from build123d import *

# Parameters (mm, degrees)
F0_W      = 75
F0_H      = 70
F0_R      = 3.3
F0_W_2    = 30
F0_H_2    = 13.5
F1_DEPTH  = 5
F2_W      = 4
F2_H      = 70
F3_DEPTH  = 55
F4_R      = 19
F4_R_2    = 2.25
F5_DEPTH  = 4
F7_W      = 65.0362595889
F7_H      = 5
F9_R      = 5
F10_DEPTH = 10
F11_R     = 6


with BuildPart() as f1:
    # F0 (on Front) → F1 (new body)
    with BuildSketch(Plane.XZ):
        Rectangle(F0_W, F0_H)
        with Locations((-31.5, -23)):
            Circle(F0_R, mode=Mode.SUBTRACT)
        with Locations((-18.5, -23)):
            Circle(F0_R, mode=Mode.SUBTRACT)
        with Locations((4.5, -10.75)):
            Rectangle(F0_W_2, F0_H_2, mode=Mode.SUBTRACT)
        with Locations((-31.5, 23)):
            Circle(F0_R, mode=Mode.SUBTRACT)
        with Locations((-18.5, 23)):
            Circle(F0_R, mode=Mode.SUBTRACT)
        with Locations((4.5, 10.75)):
            Rectangle(F0_W_2, F0_H_2, mode=Mode.SUBTRACT)
    extrude(amount=F1_DEPTH)

    # F2 (on face) → F3 (join)
    with BuildSketch(Plane.XZ.offset(5)):
        with Locations((35.5, 0)):
            Rectangle(F2_W, F2_H)
    extrude(amount=F3_DEPTH)

    # F4 (on face) → F5 (cut, through all)
    with BuildSketch(Plane.YZ.offset(37.5)):
        with Locations((-30, 0)):
            Circle(F4_R)
        with Locations((-53.5, 23.5)):
            Circle(F4_R_2)
        with Locations((-6.5, 23.5)):
            Circle(F4_R_2)
        with Locations((-6.5, -23.5)):
            Circle(F4_R_2)
        with Locations((-53.5, -23.5)):
            Circle(F4_R_2)
    extrude(amount=-F5_DEPTH, mode=Mode.SUBTRACT)

    # F7 (on line) → F8 (join, up to the next surface of F1)
    with BuildSketch(Plane(origin=(-7.3353011104, -6.1550484563, 0), x_dir=(0.6427876097, -0.7660444431, 0), z_dir=(-0.7660444431, -0.6427876097, 0))):
        with Locations((31.01032112, 32.5)):
            Rectangle(F7_W, F7_H)
        with Locations((31.01032112, -32.5)):
            Rectangle(F7_W, F7_H)
    extrude(until=Until.NEXT, dir=(0.7660444431, 0.6427876097, 0))

    # F9 (on face) → F10 (cut)
    with BuildSketch(Plane(origin=(33.5, 0, 0), x_dir=(0, -1, 0), z_dir=(-1, 0, 0))):
        with Locations((6.5, 23.5000000002)):
            Circle(F9_R)
        with Locations((6.5, -23.4999999998)):
            Circle(F9_R)
    extrude(amount=F10_DEPTH, mode=Mode.SUBTRACT)

    # F11
    f11_edges = [f1.edges().sort_by_distance(p)[0] for p in [
        (-10.5, -2.5, 17.5),
        (19.5, -2.5, 17.5),
        (19.5, -2.5, 4),
        (-10.5, -2.5, 4),
        (19.5, -2.5, -4),
        (19.5, -2.5, -17.5),
        (-10.5, -2.5, -17.5),
        (-10.5, -2.5, -4),
    ]]
    fillet(f11_edges, radius=F11_R)


solid = f1.part
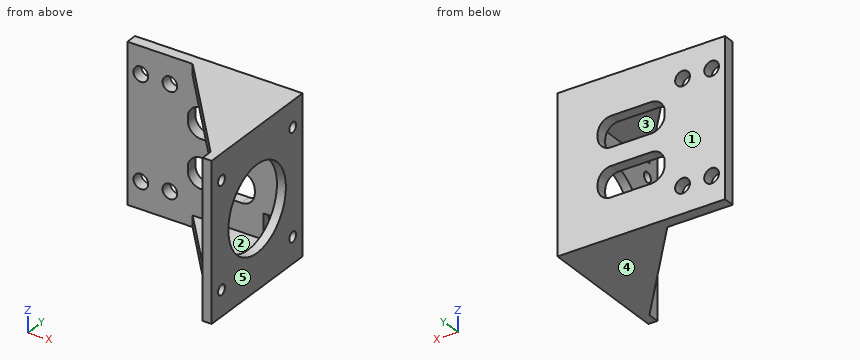
Read the model definition and answer for the solid it produces. Units are mm, in the model's axes. Face numbers are marked on the shaded views. A direction names the side the tool comes from. Give positions to 0.01 mm unless a question says otherwise; leave off trailing zeros. Loops run counter-clockwise (first coordinate to the right, second up) from the corner with the lowest first, then second, coordinate; pieces in that order, holes last. Notation, with made-up numbers: (-28, 30) -> (9, 30) arc R29 ccw to (9, 61) -> close; hole circle Ø6 at (52, 35.25). An arc over 180 degrees is marked (long way). Use a Markdown table: item, result.
Q1. Determine the mould class of the marked faces 3, 4 and 5 for opening direction Z: pulls with the +Z half, pulls with the -Z half, needs draft (parallel to the pull), parting line crosses it, or undercut.
Solved:
| item | result |
|---|---|
| face 3 | undercut |
| face 4 | pulls with the -Z half |
| face 5 | needs draft |
Q2. Find the intervals of material crossed by line 1 along Z through (x, y) = (-31.5, -2.1); line 2 along Z through (x, y) = (34.3, -6.5); line 3 along Z through (x, y) = (17, -15), in increasing order.
Solved:
| item | result |
|---|---|
| line 1 | z = -35 to -26.3, -19.7 to 19.7, 26.3 to 35 |
| line 2 | z = -35 to -25.75, -21.25 to 21.25, 25.75 to 35 |
| line 3 | z = -35 to -30, 30 to 35 |
Q3. Each of these flat-tipped pins is pushed along its axis until it touches: pin 1 (10 mm diameter, centred on x = -1.5, z = -22, fed in from -Y); pin 2 (8 mm diameter, centred on x = -2, z = -28, fed in from -Y); pin 3 (12 mm diameter, centred on y = -31.5, z = -10.5, fed in from -X); pin 4 (10 mm diameter, centred on y = -33, z = -17.5, fed in from -X). Where does it stop, or does it pass through?
Solved:
| item | result |
|---|---|
| pin 1 | stops at y = -5 |
| pin 2 | stops at y = -16.64 |
| pin 3 | passes through |
| pin 4 | stops at x = 33.5 |
Q4. Section B-B, the plane x = -31.5 is taken. Determine the outline of the cut face in (y, z).
Solved:
| item | result |
|---|---|
| outline | (-5, -35) -> (0, -35) -> (0, -26.3) -> (-5, -26.3) -> close; (-5, -19.7) -> (0, -19.7) -> (0, 19.7) -> (-5, 19.7) -> close; (-5, 26.3) -> (0, 26.3) -> (0, 35) -> (-5, 35) -> close |
Q5. Section A-A, the plane z = 0 is taken. Determine the outline of the cut face in (x, y).
Solved:
| item | result |
|---|---|
| outline | (-37.5, -5) -> (33.5, -5) -> (33.5, -11) -> (37.5, -11) -> (37.5, 0) -> (-37.5, 0) -> close; (33.5, -60) -> (37.5, -60) -> (37.5, -49) -> (33.5, -49) -> close |
Q6. Section D-D, the plane z = -15.5 is taken. Determine the outline of the cut face in (x, y).
Solved:
| item | result |
|---|---|
| outline | (-37.5, -5) -> (-8.97, -5) -> (-8.97, 0) -> (-37.5, 0) -> close; (17.97, -5) -> (33.5, -5) -> (33.5, -19.01) -> (37.5, -19.01) -> (37.5, 0) -> (17.97, 0) -> close; (33.5, -60) -> (37.5, -60) -> (37.5, -40.99) -> (33.5, -40.99) -> close |
Q7. Section C-C, the plane y = -26 is taken. Determine the outline of the cut face in (x, z), then the cut area to 3 significant figures.
Solved:
| item | result |
|---|---|
| outline | (9.32, -35) -> (37.5, -35) -> (37.5, -18.57) -> (33.5, -18.57) -> (33.5, -30) -> (9.32, -30) -> close; (9.32, 30) -> (33.5, 30) -> (33.5, 18.57) -> (37.5, 18.57) -> (37.5, 35) -> (9.32, 35) -> close |
| area | 373 mm^2 |
Q8. A tool of negligible diameter and unlimited length cuts with its end or side. For the marked faces 1 and 2, from which of +Z, -Z, +X, -X, +Y, -Y can it reach the whole face along a straight path? Write none if from no direction.
Solved:
| item | result |
|---|---|
| face 1 | +Z, -Z, +X, -X, +Y |
| face 2 | -X, -Y |
